Source: CAD feature listing. Evaluate the final solid. Frame: model axes, mm. Face numbers are marked on the shaded views. A direction names the side the tool comes from. Coordinates: 2 decimals unless noted, no trailing zeros. Write each loop counter-clockwise with the first axis right and the second up, starting at its lowest first coordinate (ties: lowest second). Pieces come first, ordered by that corner, then holes. Notation, with made-up numbers: (8.25, 49.5) - (65.25, 49.5) arc R27 ccw to (65.25, 66.5) - close; hole circle Ø10 at (-24, -1.75). An arc over 180 degrees is marked (long way). One line per item, written item: value.
from build123d import *

# Parameters (mm, degrees)
SKETCH1_W           = 200
SKETCH1_H           = 116
BOSS_EXTRUDE1_DEPTH = 90
SHELL1_T            = -2
SKETCH2_R           = 35
CUT_EXTRUDE1_DEPTH  = 10
SKETCH3_R           = 30
CUT_EXTRUDE2_DEPTH  = 10


with BuildPart() as part:
    # Sketch1 → Boss-Extrude1 (new body)
    with BuildSketch(Plane.XY):
        with Locations((-123.252218957, -176.05574429)):
            Rectangle(SKETCH1_W, SKETCH1_H)
    extrude(amount=BOSS_EXTRUDE1_DEPTH)

    # Shell1
    shell1_openings = [part.faces().sort_by_distance(p)[0] for p in [
        (-123.252218957, -176.05574429, 0),
    ]]
    offset(amount=SHELL1_T, openings=shell1_openings, kind=Kind.INTERSECTION)

    # Sketch2 → Cut-Extrude1 (cut)
    with BuildSketch(Plane(origin=(0, 0, 88), x_dir=(-1, 0, 0), z_dir=(0, 0, -1))):
        with Locations((83.252218957, -176.05574429)):
            Circle(SKETCH2_R)
    extrude(amount=-CUT_EXTRUDE1_DEPTH, mode=Mode.SUBTRACT)

    # Sketch3 → Cut-Extrude2 (cut)
    with BuildSketch(Plane(origin=(0, -118.05574429, 0), x_dir=(1, 0, 0), z_dir=(0, 1, 0))):
        with Locations(Location((-171.255446698, -45.579189532, 0), (0, 0, 180))):
            Circle(SKETCH3_R)
    extrude(amount=-CUT_EXTRUDE2_DEPTH, mode=Mode.SUBTRACT)


solid = part.part
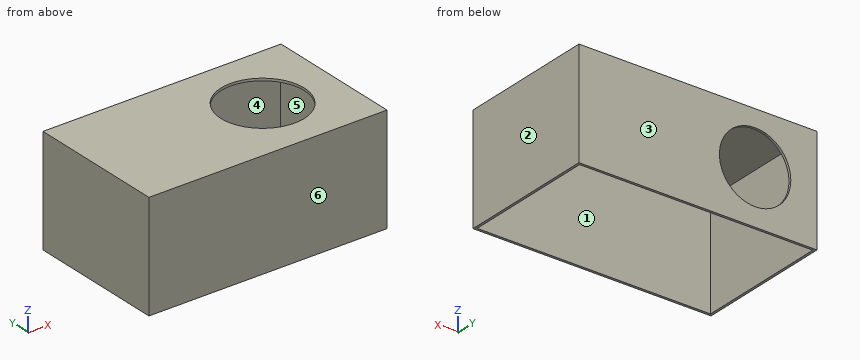
1) Draft query along Y for the marked faces 1, 2, 3 and 4. Return one class per face: released by +Y, released by -Y, zero draft, split by the parting line, or undercut.
Values found:
face 1: undercut
face 2: zero draft
face 3: released by +Y
face 4: undercut
2) Material intervals for line 1 (Y direction, x = -139.5, z = 26.5); line 2 (X direction, y = -220, z = 69); line 3 (Z direction, x = -121.5, y = -150.5), sorted ascending.
Values found:
line 1: -234.06 to -232.06, -120.06 to -118.06
line 2: -223.25 to -221.25, -25.25 to -23.25
line 3: 88 to 90
3) Contact query for a flat-ended pin moving along its axis: P1, Ø6, axis at x = -162, y = -171, coming from the -Z side. Output: stop coordinate, or through.
Values found:
P1: z = 88
4) Reachability of the marked faces 5 and 6 from +Z, -Z, +X, -X, +Y, -Y: full face, straight path, thin tool, end or side. Return the list, or none.
Values found:
face 5: -Z
face 6: +Z, -Z, +X, -X, -Y
5) Section query D-D on x = -104. Output: boundary loops of the cut face in (y, z).
Values found:
outline: (-234.06, 0) - (-232.06, 0) - (-232.06, 88) - (-204.24, 88) - (-204.24, 90) - (-234.06, 90) - close; (-147.87, 88) - (-120.06, 88) - (-120.06, 0) - (-118.06, 0) - (-118.06, 90) - (-147.87, 90) - close
6) Section query C-C on x = -137. Output: boundary loops of the cut face in (y, z), then the cut area to 3 significant figures.
Values found:
outline: (-234.06, 0) - (-232.06, 0) - (-232.06, 88) - (-120.06, 88) - (-120.06, 0) - (-118.06, 0) - (-118.06, 90) - (-234.06, 90) - close
area: 584 mm2
7) Section query B-B on z = 82.5. Output: boundary loops of the cut face in (x, y), then the cut area to 3 significant figures.
Values found:
outline: (-223.25, -234.06) - (-23.25, -234.06) - (-23.25, -118.06) - (-223.25, -118.06) - close; hole (-221.25, -232.06) - (-25.25, -232.06) - (-25.25, -120.06) - (-221.25, -120.06) - close
area: 1,250 mm2
8) Section query A-A on y = -168. Output: boundary loops of the cut face in (x, z).
Values found:
outline: (-223.25, 0) - (-221.25, 0) - (-221.25, 88) - (-117.31, 88) - (-117.31, 90) - (-223.25, 90) - close; (-49.19, 88) - (-25.25, 88) - (-25.25, 0) - (-23.25, 0) - (-23.25, 90) - (-49.19, 90) - close
